Work out the finished part from the listing and answer in its coordinate system (mm). A direction names the side the tool comes from. Coordinates: 2 decimals unless noted, no trailing zeros. Order: outer loops, then holes, each group sorted by start corner. A loop starts at its lowest first (then second) coordinate and runs counter-clockwise, first axis right, second up. Notation, with made-up numbers: (-38.75, -2.75) -> (2.25, -2.75) arc R30 ccw to (2.25, 28.25) -> close; hole circle Ø3 at (-39, 25). An arc over 180 degrees is marked (long way). Use one line per item in the form item = value.
from build123d import *

# Parameters (mm, degrees)
SKETCH_1_R          = 16
EXTRUDE_1_DEPTH     = 7
SKETCH_2_R          = 14.85
EXTRUDE_2_DEPTH     = 16
SKETCH_3_R          = 1.6
CUT_EXTRUDE_1_DEPTH = 33.26453161
SKETCH_4_R          = 2.9
CUT_EXTRUDE_2_DEPTH = 33.26453161


with BuildPart() as part:
    # 草图1 → 凸台-拉伸1 (new body)
    with BuildSketch(Plane(origin=(0, 0, 0), x_dir=(1, 0, 0), z_dir=(0, 1, 0))):
        with Locations(Location((0, 0, 0), (0, 0, 270))):
            Circle(SKETCH_1_R)
    extrude(amount=EXTRUDE_1_DEPTH)

    # 草图2 → 凸台-拉伸2 (add)
    with BuildSketch(Plane(origin=(0, 7, 0), x_dir=(1, 0, 0), z_dir=(0, 1, 0))):
        with Locations(Location((0, 0, 0), (0, 0, 270))):
            Circle(SKETCH_2_R)
    extrude(amount=EXTRUDE_2_DEPTH)

    # 草图3 → 切除-拉伸1 (cut, through all)
    with BuildSketch(Plane(origin=(0, 23, 0), x_dir=(1, 0, 0), z_dir=(0, 1, 0))):
        with Locations(Location((0, 12.5, 0), (0, 0, 270))):
            Circle(SKETCH_3_R)
        with Locations(Location((10.825317547, 6.25, 0), (0, 0, 270))):
            Circle(SKETCH_3_R)
        with Locations(Location((10.825317547, -6.25, 0), (0, 0, 270))):
            Circle(SKETCH_3_R)
        with Locations(Location((0, -12.5, 0), (0, 0, 270))):
            Circle(SKETCH_3_R)
        with Locations(Location((-10.825317547, -6.25, 0), (0, 0, 270))):
            Circle(SKETCH_3_R)
        with Locations(Location((-10.825317547, 6.25, 0), (0, 0, 270))):
            Circle(SKETCH_3_R)
    extrude(amount=-CUT_EXTRUDE_1_DEPTH, mode=Mode.SUBTRACT)

    # 草图4 → 切除-拉伸2 (cut, through all)
    with BuildSketch(Plane.XZ):
        with Locations((8.75, 15.155444566)):
            Circle(SKETCH_4_R)
        with Locations((17.5, 0)):
            Circle(SKETCH_4_R)
        with Locations((8.75, -15.155444566)):
            Circle(SKETCH_4_R)
        with Locations((-8.75, -15.155444566)):
            Circle(SKETCH_4_R)
        with Locations((-17.5, 0)):
            Circle(SKETCH_4_R)
        with Locations((-8.75, 15.155444566)):
            Circle(SKETCH_4_R)
    extrude(amount=-CUT_EXTRUDE_2_DEPTH, mode=Mode.SUBTRACT)


solid = part.part
(1) Each of these flat-tipped pins is pushed along its axis until it touches: P1, Ø2.5, axis at x = 10.83, z = 6.25, coming from the -Y side; P2, Ø5, axis at x = -6, y = 19, coming from the -Z side; P3, Ø4, axis at y = 9.5, z = -7, coming from the +X side; P4, Ø1, axis at y = 16.5, z = -11, coming from the -X side. Where does it stop, or does it pass through?
Data:
P1 = through
P2 = -14.43
P3 = 13.98
P4 = -10.5
(2) Section A-A on x = 0 is taken. Write down the section's boundary in (y, z).
Data:
outline = (0, -16) -> (7, -16) -> (7, -14.85) -> (23, -14.85) -> (23, -14.1) -> (0, -14.1) -> close; (0, -10.9) -> (23, -10.9) -> (23, 10.9) -> (0, 10.9) -> close; (0, 14.1) -> (23, 14.1) -> (23, 14.85) -> (7, 14.85) -> (7, 16) -> (0, 16) -> close
(3) Section C-C on y = 13.75 is taken. Write down the section's boundary in (x, z), plus the area to 3 significant figures.
Data:
outline = (-14.81, -1.08) arc R14.85 ccw to (-8.34, -12.28) arc R2.9 cw to (-6.47, -13.37) arc R14.85 ccw to (6.47, -13.37) arc R2.9 cw to (8.34, -12.28) arc R14.85 ccw to (14.81, -1.08) arc R2.9 cw to (14.81, 1.08) arc R14.85 ccw to (8.34, 12.28) arc R2.9 cw to (6.47, 13.37) arc R14.85 ccw to (-6.47, 13.37) arc R2.9 cw to (-8.34, 12.28) arc R14.85 ccw to (-14.81, 1.08) arc R2.9 cw to start; hole circle Ø3.2 at (-10.83, -6.25); hole circle Ø3.2 at (-10.83, 6.25); hole circle Ø3.2 at (0, -12.5); hole circle Ø3.2 at (0, 12.5); hole circle Ø3.2 at (10.83, -6.25); hole circle Ø3.2 at (10.83, 6.25)
area = 642 mm²
(4) The mould has two halves that part along X. Classify faces 4 (the cylindrical face through (13.8, 3.5, 8.1)), 5 (the flat face through (0, 7, 15)), 6 (the cylindrical face through (7.27, 8.78, 12.66)): released by +X, released by -X, zero draft, split by the parting line, or undercut.
Data:
face_4 = released by +X
face_5 = zero draft
face_6 = undercut
(5) Section D-D on z = 11.5 is taken. Write down the section's boundary in (x, y).
Data:
outline = (-11.12, 0) -> (-1.25, 0) -> (-1.25, 23) -> (-9.4, 23) -> (-9.4, 7) -> (-11.12, 7) -> close; (1.25, 0) -> (11.12, 0) -> (11.12, 7) -> (9.4, 7) -> (9.4, 23) -> (1.25, 23) -> close
(6) Straight lines are drawn through the part: line 1 along X through (y, z) = (12, -6.25); line 2 along Z through (x, y) = (-1, 9); line 3 along X through (y, z) = (18.5, -6). For each, find the intervals that lie inside material, in ascending order.
Data:
line_1 = -13.47 to -12.43, -9.23 to 9.23, 12.43 to 13.47
line_2 = -14.82 to -13.75, -11.25 to 11.25, 13.75 to 14.82
line_3 = -13.58 to -12.41, -9.24 to 9.24, 12.41 to 13.58
(7) Section B-B on z = 6.25 is taken. Write down the section's boundary in (x, y).
Data:
outline = (-14.73, 0) -> (-12.43, 0) -> (-12.43, 23) -> (-13.47, 23) -> (-13.47, 7) -> (-14.73, 7) -> close; (-9.23, 0) -> (9.23, 0) -> (9.23, 23) -> (-9.23, 23) -> close; (12.43, 0) -> (14.73, 0) -> (14.73, 7) -> (13.47, 7) -> (13.47, 23) -> (12.43, 23) -> close
(8) Which of the six approach directions +Z, -Z, +X, -X, +Y, -Y give full straight-line access (tool end or side, diameter ignored) to faces 1 (the cylindrical face through (-12.91, 14.89, 7.34)), 2 (the flat face through (13, 7, 8)), 3 (the cylindrical face through (12.91, 14.89, -7.34))?
Data:
face_1 = +Z, -X, +Y
face_2 = +Z, +X, +Y
face_3 = -Z, +X, +Y
